Verification items for this drawing (mm, ordinates from the low corner). Round coordinates to 2 decimals unless told otherwise and drop trailing zeros. Loops run counter-clockwise (first coordinate to the right, second up) from the corner with the lowest first, then second, coordinate; pieces in that order, holes last. Notation, with made-up numbers: (10.25, -26.5) - (30.25, -26.5) arc R31 ccw to (30.25, -1.5) - close; hole circle Ø6 at (6, 45.5). An arc over 180 degrees is marked (long way). Put each result on its own line as item: value.
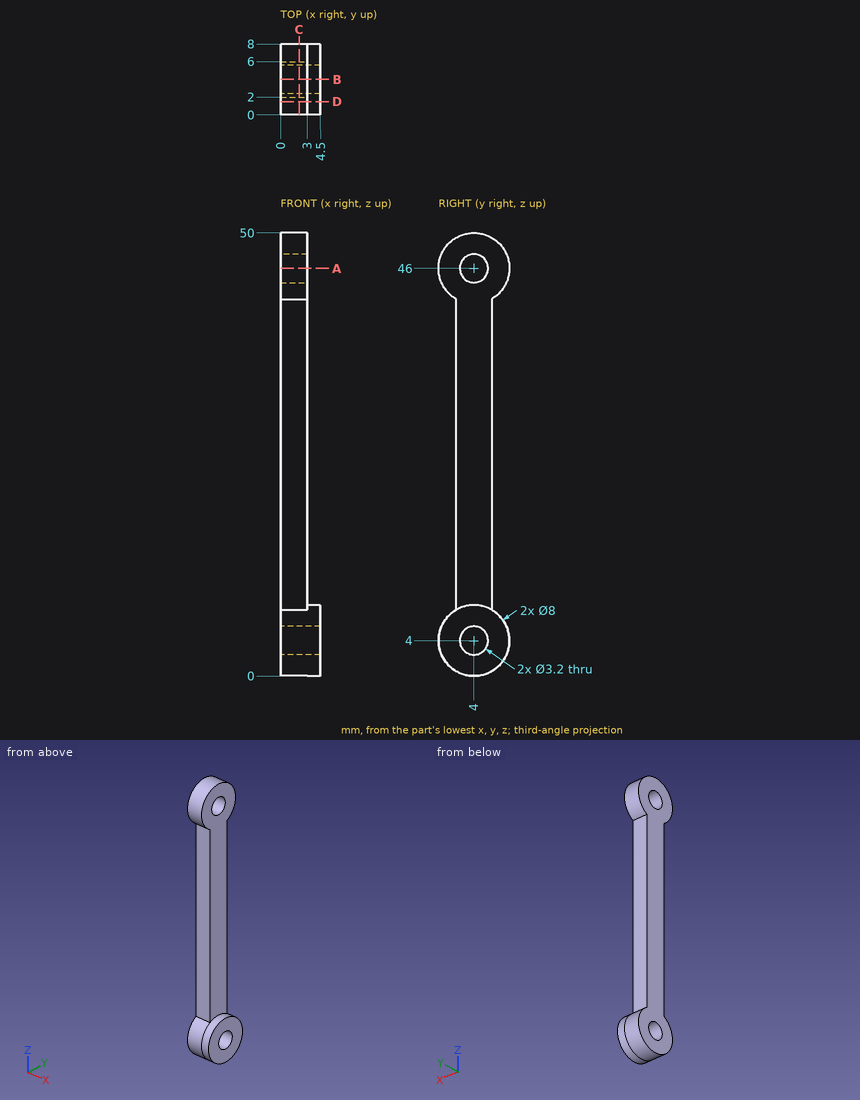
Item 1: Section check C-C on x = 2.1. Enter the section's corners in (y, z), then the cut area to 3 significant figures.
Filled sheet:
outline: (2, 7.46) arc R4 ccw (long way) to (6, 7.46) - (6, 42.54) arc R4 ccw (long way) to (2, 42.54) - close; hole circle Ø3.2 at (4, 4); hole circle Ø3.2 at (4, 46)
area: 222 mm²
Item 2: Section check D-D on y = 1.5. Enter the section's corners in (x, z).
Filled sheet:
outline: (0, 0.88) - (4.5, 0.88) - (4.5, 7.12) - (0, 7.12) - close; (0, 42.88) - (3, 42.88) - (3, 49.12) - (0, 49.12) - close
Item 3: Thickness scan on line 1 (Y direction, x = 1.7, z = 4); line 2 (X direction, y = 2.5, z = 41.5); line 3 (Y direction, x = 2.4, z = 30.5). Record the ranges inside material, lowest first. Write a range as from..to.
Filled sheet:
line 1: 0..2.4, 5.6..8
line 2: 0..3
line 3: 2..6
Item 4: Go/stop test with flat-tipped pins: pin 1 (3 mm diameter, centred on y = 6, z = 32.5, fed in from +X); pin 2 (2.5 mm diameter, centred on x = 1.5, z = 23, fed in from -Y); pin 3 (1.5 mm diameter, centred on x = 2.5, y = 3.5, fed in from -Z); pin 4 (1.5 mm diameter, centred on x = 1.5, z = 17.5, fed in from +Y). Record where each tip stops, or that it passes through.
Filled sheet:
pin 1: x = 3
pin 2: y = 2
pin 3: z = 0
pin 4: y = 6
Item 5: Section check B-B on y = 4. Enter the section's corners in (x, z), then the cut area to 3 significant figures.
Filled sheet:
outline: (0, 0) - (4.5, 0) - (4.5, 2.4) - (0, 2.4) - close; (0, 5.6) - (4.5, 5.6) - (4.5, 8) - (3, 8) - (3, 44.4) - (0, 44.4) - close; (0, 47.6) - (3, 47.6) - (3, 50) - (0, 50) - close
area: 138 mm²
Item 6: Section check A-A on z = 46. Enter the section's corners in (x, y), then the cut area to 3 significant figures.
Filled sheet:
outline: (0, 0) - (3, 0) - (3, 2.4) - (0, 2.4) - close; (0, 5.6) - (3, 5.6) - (3, 8) - (0, 8) - close
area: 14.4 mm²
